Verification items for the finished model (mm, model axes). Face numbers are marked on the shaded views. A direction names the side the tool comes from. Coordinates: 2 decimals unless noted, no trailing zeros. Write each loop counter-clockwise with the first axis right and the second up, starting at its lowest first coordinate (ties: lowest second). Pieces come first, ordered by that corner, then holes. Notation, with made-up numbers: M 53.25,63 L 99.25,63 A19 ccw 99.25,85 Z; hole C 40.25,80.5 d6. An arc over 180 degrees is marked long. Answer in a Markdown table with one row per item.
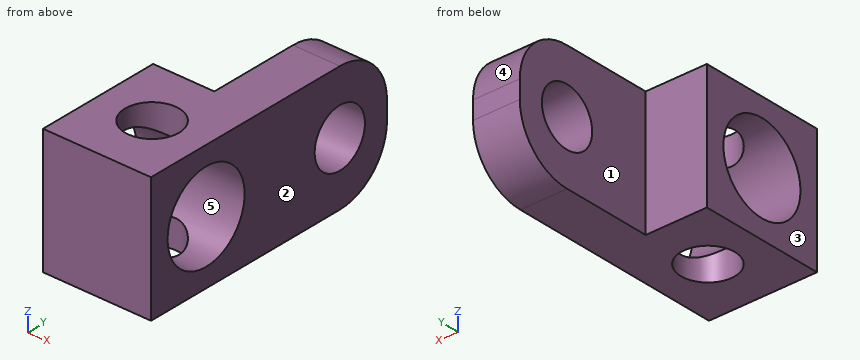
from build123d import *

# Parameters (mm, degrees)
F0_W      = 6
F0_H      = 15
F1_DEPTH  = 7
F2_W      = 3.4
F2_H      = 8
F3_DEPTH  = 25
F4_R      = 3
F5_R      = 2.45
F6_DEPTH  = 25
F7_R      = 1.6
F8_DEPTH  = 25
F9_R      = 1.5
F10_DEPTH = 25


with BuildPart() as f1:
    # F0 (on Top) → F1 (new body)
    with BuildSketch(Plane.XY):
        with Locations((3, 7.5)):
            Rectangle(F0_W, F0_H)
    extrude(amount=-F1_DEPTH)

    # F2 (on face) → F3 (cut)
    with BuildSketch(Plane.XY):
        with Locations((1.7, 11)):
            Rectangle(F2_W, F2_H)
    extrude(amount=-F3_DEPTH, mode=Mode.SUBTRACT)

    # F4
    f4_edges = [f1.edges().sort_by_distance(p)[0] for p in [
        (4.7, 15, 0),
        (4.7, 15, -7),
    ]]
    fillet(f4_edges, radius=F4_R)

    # F5 (on face) → F6 (cut)
    with BuildSketch(Plane(origin=(0, 0, 0), x_dir=(0, -1, 0), z_dir=(-1, 0, 0))):
        with Locations((-3.5, -3.5)):
            Circle(F5_R)
    extrude(amount=-F6_DEPTH, mode=Mode.SUBTRACT)

    # F7 (on face) → F8 (cut)
    with BuildSketch(Plane(origin=(3.4, 0, 0), x_dir=(0, -1, 0), z_dir=(-1, 0, 0))):
        with Locations((-12, -3.5)):
            Circle(F7_R)
    extrude(amount=-F8_DEPTH, mode=Mode.SUBTRACT)

    # F9 (on face) → F10 (cut)
    with BuildSketch(Plane(origin=(0, 0, -7), x_dir=(1, 0, 0), z_dir=(0, 0, -1))):
        with Locations((3, -3.5)):
            Circle(F9_R)
    extrude(amount=-F10_DEPTH, mode=Mode.SUBTRACT)


solid = f1.part
1) Thickness scan on L1, parallel to Y at x = 3, z = -0.5; L2, parallel to Z at x = 4.5, y = 12; L3, parallel to Y at x = 4.5, z = -4.25. Record the ranges inside material, lowest first. Write a range as [from, to].
Response values:
| item | result |
|---|---|
| L1 | y = [0, 2], [5, 7] |
| L2 | z = [-7, -5.1], [-1.9, 0] |
| L3 | y = [0, 1.17], [5.83, 10.59], [13.41, 14.99] |
2) Tool access check on the marked faces 1 and 2. Record the directions out of +Z, -Z, +X, -X, +Y, -Y that give a thin tool (end or side, any length) a straight path to the whole face; none if there is none.
Response values:
| item | result |
|---|---|
| face 1 | +Z, -Z, -X, +Y |
| face 2 | +Z, -Z, +X, +Y, -Y |
3) Sectioned sample at A-A (y = 3.5). Record the cut outline in (x, z).
Response values:
| item | result |
|---|---|
| outline | M 0,-7 L 1.5,-7 L 1.5,-5.95 L 0,-5.95 Z; M 0,-1.05 L 1.5,-1.05 L 1.5,0 L 0,0 Z; M 4.5,-7 L 6,-7 L 6,-5.95 L 4.5,-5.95 Z; M 4.5,-1.05 L 6,-1.05 L 6,0 L 4.5,0 Z |
4) Sectioned sample at C-C (x = 3). Record the cut outline in (y, z), then the cut area to 3 significant figures.
Response values:
| item | result |
|---|---|
| outline | M 0,-7 L 2,-7 L 2,-5.44 A2.45 cw 2,-1.56 L 2,0 L 0,0 Z; M 5,-7 L 7,-7 L 7,0 L 5,0 L 5,-1.56 A2.45 cw 5,-5.44 Z |
| area | 22.9 mm² |
5) Sectioned sample at D-D (x = 0.5). Record the cut outline in (y, z), then the cut area to 3 significant figures.
Response values:
| item | result |
|---|---|
| outline | M 0,-7 L 7,-7 L 7,0 L 0,0 Z; hole C 3.5,-3.5 d4.9 |
| area | 30.1 mm² |
6) Depth check by flat-ended pin: pin 1 (1.7 mm diameter, centred on x = 2.5, z = -2, fed in from +Y); pin 2 (4 mm diameter, centred on y = 11.5, z = -3, fed in from +X); pin 3 (1 mm diameter, centred on x = 3.5, y = 13, fed in from -Z). Enter the tip coordinate at first touch or a pass-through.
Response values:
| item | result |
|---|---|
| pin 1 | stops at y = 7 |
| pin 2 | stops at x = 6 |
| pin 3 | stops at z = -6.96 |
7) Sectioned sample at B-B (z = -3.5). Record the cut outline in (x, y).
Response values:
| item | result |
|---|---|
| outline | M 0,0 L 6,0 L 6,1.05 L 0,1.05 Z; M 0,5.95 L 6,5.95 L 6,10.4 L 3.4,10.4 L 3.4,7 L 0,7 Z; M 3.4,13.6 L 6,13.6 L 6,15 L 3.4,15 Z |
8) Release check for a two-part mould opening along Y. For the marked faces 3, 4 and 5 record: +Y half, -Y half, draft (parallel to the pull), parting line (faces both ways), or undercut.
Response values:
| item | result |
|---|---|
| face 3 | draft |
| face 4 | +Y half |
| face 5 | undercut |
